Design review of the part built by this model. Coordinates are the model's own, in mm. Coordinates: 2 decimals unless noted, no trailing zeros. Write each loop counter-clockwise with the first axis right and the second up, starting at its lowest first coordinate (ties: lowest second). Pieces come first, ordered by that corner, then holes. Notation, with made-up numbers: (42.25, -36.5) -> (67.25, -36.5) arc R16 cw to (67.25, -5.5) -> close; hole circle Ø6 at (32.5, 23). An arc over 180 degrees is marked (long way). Answer in a Markdown table with one row per item. Add a question column.
Item 1: Clearance check with flat-ended pins moving along their axes: P1, Ø5, axis at y = 7, z = -117.5, coming from the -X side; P2, Ø3, axis at x = -1, y = 5, coming from the +Z side; P3, Ø2, axis at x = -3, y = 6, coming from the +Z side; P4, Ø1, axis at x = -2.5, y = 7.5, coming from the -Z side. State where each tip first meets the part, or that it passes through.
Item 2: Take a section at B-B, the plane x = -4.5. Write out the cut boundary in (y, z), and give its area (3 significant figures).
Item 3: To check wall thickness, follow line 1 (X direction, y = 1.5, z = -75); line 2 (X direction, y = 9, z = -69); line 3 (Z direction, x = -2.5, y = 9.25). State the ranges of each line that lie inside material, in increasing order.
Item 4: Take a section at C-C, the plane z = -85. Write out the cut boundary in (x, y).
Item 5: Take a section at A-A, the plane y = 7.5. Write out the cut boundary in (x, z).
Autodesk Inventor part; units mm, degrees
ref_plane "YZ Plane" through (0, 0, 0) normal (1, 0, 0) x (0, 1, 0)
ref_plane "XZ Plane" through (0, 0, 0) normal (0, 1, 0) x (-1, 0, 0)
ref_plane "XY Plane" through (0, 0, 0) normal (0, 0, 1) x (1, 0, 0)
sketch "Sketch1" plane through (0, 0, 0) normal (0, 1, 0) x (-1, 0, 0)
  line L0 (0, 0) -> (0, -141.096) construction
  line L1 (-3, 0) -> (-3, -141.096)
  line L2 (3, -141.096) -> (3, 0)
  arc A0 (3, 0) -> (-3, 0) centre (0, 0) ccw
  arc A1 (-3, -141.096) -> (3, -141.096) centre (0, -141.096) ccw
  circle A2 centre (0, 0) radius 1.5
  circle A3 centre (0, -141.096) radius 1.5
  arc A4 (-3, -141.096) -> (-3, 0) centre (-598.838, -70.548) ccw
  arc A5 (3, -141.096) -> (3, 0) centre (-592.838, -70.548) ccw
  point P0 (0, -70.548)
  dimension "d0" = 6
  dimension "d1" = 141.096
  dimension "d2" = 3
  dimension "d3" = 3
  dimension "d10" = 600
  dimension "d11" = 600
extrude "Extrusion1" add sketch "Sketch1" along normal blind 10 contours A0 L2 A1 A4 | A5 L2
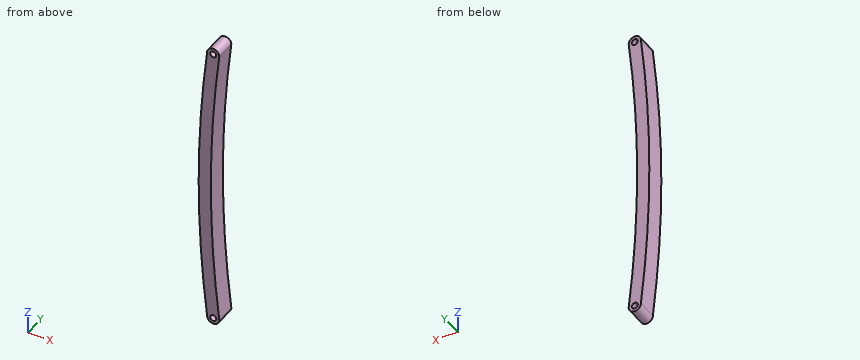
Answers:
| question | item | result |
|---|---|---|
| 1 | P1 | stops at x = -5.51 |
| 1 | P2 | stops at z = 3 |
| 1 | P3 | stops at z = 2.24 |
| 1 | P4 | stops at z = -143.33 |
| 2 | outline | (0, -127) -> (10, -127) -> (10, -14.09) -> (0, -14.09) -> close |
| 2 | area | 1,130 mm^2 |
| 3 | line 1 | x = -7.15 to -1.15 |
| 3 | line 2 | x = -7.16 to -1.16 |
| 3 | line 3 | z = -142.75 to 1.66 |
| 4 | outline | (-6.99, 0) -> (-0.99, 0) -> (-0.99, 10) -> (-6.99, 10) -> close |
| 5 | outline | (-3, -141.1) arc R3 ccw to (3, -141.1) arc R600 cw to (3, 0) arc R3 ccw to (-3, 0) arc R600 ccw to start; hole circle Ø3 at (0, -141.1); hole circle Ø3 at (0, 0) |
